from build123d import *

# Parameters (mm, degrees)
SKETCH_R     = 26
PAD_DEPTH    = 40
SKETCH001_R  = 3.25
POCKET_DEPTH = 68.001


with BuildPart() as part:
    # Sketch → Pad (new body)
    with BuildSketch(Plane.XY):
        Polygon((-45, 0), (45, 0), (45, 17), (42.5, 22), (42.5, 54), (27.5, 54), (13.5, 68), (-13.5, 68), (-27.5, 54), (-42.5, 54), (-42.5, 22), (-45, 17), align=None)
        with Locations((0, 34)):
            Circle(SKETCH_R, mode=Mode.SUBTRACT)
    extrude(amount=PAD_DEPTH)

    # Sketch001 (on Face1 of Pad) → Pocket (cut, through all)
    with BuildSketch(Plane.XZ):
        with Locations((-35, 30)):
            Circle(SKETCH001_R)
        with Locations((-35, 10)):
            Circle(SKETCH001_R)
        with Locations((35, 10)):
            Circle(SKETCH001_R)
        with Locations((35, 30)):
            Circle(SKETCH001_R)
    extrude(amount=-POCKET_DEPTH, mode=Mode.SUBTRACT)


solid = part.part
Source: CAD feature listing. Evaluate the final solid. Frame: model axes, mm. A direction names the side the tool comes from. Coordinates: 2 decimals unless noted, no trailing zeros. Loops run counter-clockwise (first coordinate to the right, second up) from the corner with the lowest first, then second, coordinate; pieces in that order, holes last. Notation, with made-up numbers: (9, 44) - (45, 44) arc R34 ccw to (45, 77) - close; hole circle Ø4 at (-19, 34). An arc over 180 degrees is marked (long way). Return JSON: item names as keys, results as strings.
Q1. Contact query for flat-ended pins moving along their axis: P1, Ø4.5, axis at x = 37, z = 20.5, coming from the +Y side; P2, Ø8, axis at y = 38.5, z = 26, coming from the -X side; P3, Ø9.5, axis at y = 30, z = 29, coming from the +X side. Output: stop coordinate, or through.
Results:
{"P1": "y = 54", "P2": "x = -42.5", "P3": "x = 42.5"}
Q2. Material intervals for line 1 along Z through (x, y) = (35, 38.5); line 2 along X through (y, z) = (36, 12); line 3 along Z through (x, y) = (32.5, 21), sorted ascending.
Results:
{"line 1": "0 to 6.75, 13.25 to 26.75, 33.25 to 40", "line 2": "-42.5 to -37.56, -32.44 to -25.92, 25.92 to 32.44, 37.56 to 42.5", "line 3": "0 to 7.92, 12.08 to 27.92, 32.08 to 40"}
Q3. Section A-A, the plane y = 10. Return loops of the section in (x, z), plus the area to 3 significant figures.
Results:
{"outline": "(-45, 0) - (-10, 0) - (-10, 40) - (-45, 40) - close; (10, 0) - (45, 0) - (45, 40) - (10, 40) - close; hole circle Ø6.5 at (-35, 10); hole circle Ø6.5 at (-35, 30); hole circle Ø6.5 at (35, 10); hole circle Ø6.5 at (35, 30)", "area": "2,670 mm2"}
Q4. Access query for faces 1 (the flat face through (35, 54, 20)), 2 (the flat face through (-45, 9, 20)), 3 (the flat face through (-42.5, 38, 20)). Directions: +Z, -Z, +X, -X, +Y, -Y. A direction counts if a zero-diameter tool reaches every point of the face in a straight line with its end or side. Return the directions, or none.
Results:
{"face 1": "+Z, -Z, +X, +Y", "face 2": "+Z, -Z, -X, +Y, -Y", "face 3": "+Z, -Z, -X, +Y"}
Q5. Section D-D, the plane x = 35. Return loops of the section in (y, z).
Results:
{"outline": "(0, 0) - (54, 0) - (54, 6.75) - (0, 6.75) - close; (0, 13.25) - (54, 13.25) - (54, 26.75) - (0, 26.75) - close; (0, 33.25) - (54, 33.25) - (54, 40) - (0, 40) - close"}
Q6. Mould query, pull axis Z, two halves, no side actions, for faces 4 (the flat face through (20.6, 60.9, 19.7)), 5 (the cylindrical face through (36.5, 26.622, 27.117)), 6 (the flat face through (-1, 4, 40)). Classes: released by +Z, released by -Z, zero draft, split by the parting line, or undercut.
Results:
{"face 4": "zero draft", "face 5": "undercut", "face 6": "released by +Z"}
Q7. Section B-B, the plane z = 10. Return loops of the section in (x, y), plus the area to 3 significant figures.
Results:
{"outline": "(-45, 0) - (-38.25, 0) - (-38.25, 54) - (-42.5, 54) - (-42.5, 22) - (-45, 17) - close; (-31.75, 0) - (31.75, 0) - (31.75, 54) - (27.5, 54) - (13.5, 68) - (-13.5, 68) - (-27.5, 54) - (-31.75, 54) - close; (38.25, 0) - (45, 0) - (45, 17) - (42.5, 22) - (42.5, 54) - (38.25, 54) - close; hole circle Ø52 at (0, 34)", "area": "2,440 mm2"}
Q8. Section C-C, the plane x = -10. Return loops of the section in (y, z).
Results:
{"outline": "(0, 0) - (10, 0) - (10, 40) - (0, 40) - close; (58, 0) - (68, 0) - (68, 40) - (58, 40) - close"}
